from build123d import *

# Parameters (mm, degrees)
BOX063_W                   = 4
BOX063_H                   = 1.6
BOX063_DEPTH               = 0.6
CYLINDER043_R              = 1.5
CYLINDER043_DEPTH          = 0.6
CYLINDER042_R              = 2.2
CYLINDER042_DEPTH          = 0.6
BOX064_W                   = 3.6
BOX064_H                   = 0.8
BOX064_DEPTH               = 0.6
FUSION040_PLACEMENT_ANGLE  = 90
BOX061_W                   = 1.5
BOX061_H                   = 0.5
BOX061_DEPTH               = 3
BOX066_W                   = 1.5
BOX066_H                   = 0.5
BOX066_DEPTH               = 3
BOX060_W                   = 0.5
BOX060_H                   = 6
BOX060_DEPTH               = 1
BOX068_W                   = 52
BOX068_H                   = 6
BOX068_DEPTH               = 12
CYLINDER045_R              = 1.3
CYLINDER045_DEPTH          = 8
CYLINDER037_R              = 1.3
CYLINDER037_DEPTH          = 8
CYLINDER044_R              = 1.3
CYLINDER044_DEPTH          = 8
CYLINDER040_R              = 1.3
CYLINDER040_DEPTH          = 8
CYLINDER041_R              = 3
CYLINDER041_DEPTH          = 9.5
CYLINDER039_R              = 3
CYLINDER039_DEPTH          = 9.5
CYLINDER046_R              = 3
CYLINDER046_DEPTH          = 9.5
CYLINDER038_R              = 3
CYLINDER038_DEPTH          = 9.5
BOX069_W                   = 90
BOX069_H                   = 60
BOX069_DEPTH               = 1.6
BOX059_W                   = 1.5
BOX059_H                   = 5
BOX059_DEPTH               = 8.5
BOX070_W                   = 2
BOX070_H                   = 2
BOX070_DEPTH               = 2
BOX062_W                   = 2
BOX062_H                   = 2
BOX062_DEPTH               = 2
BOX065_W                   = 2
BOX065_H                   = 2
BOX065_DEPTH               = 2
BOX067_W                   = 2
BOX067_H                   = 2
BOX067_DEPTH               = 2
CHAMFER007_SIZE            = 0.6
CHAMFER007_PLACEMENT_ANGLE = 180


with BuildPart() as obj1:
    # Box063 → Box063 (new body)
    with BuildSketch(Plane(origin=(0, -0.8, 0), x_dir=(1, 0, 0), z_dir=(0, 0, 1))):
        with Locations((2, 0.8)):
            Rectangle(BOX063_W, BOX063_H)
    extrude(amount=BOX063_DEPTH)


with BuildPart() as zylinder042:
    # Cylinder043 → Cylinder043 (new body)
    with BuildSketch(Plane.XY):
        Circle(CYLINDER043_R)
    extrude(amount=CYLINDER043_DEPTH)


with BuildPart() as off:
    # Cylinder042 → Cylinder042 (new body)
    with BuildSketch(Plane.XY):
        Circle(CYLINDER042_R)
    extrude(amount=CYLINDER042_DEPTH)

    # Cut026: cut Zylinder042
    add(zylinder042.part, mode=Mode.SUBTRACT)

    # Cut023: cut obj1
    add(obj1.part, mode=Mode.SUBTRACT)


with BuildPart() as obj2:
    # Box064 → Box064 (new body)
    with BuildSketch(Plane(origin=(0, -0.4, 0), x_dir=(1, 0, 0), z_dir=(0, 0, 1))):
        with Locations((1.8, 0.4)):
            Rectangle(BOX064_W, BOX064_H)
    extrude(amount=BOX064_DEPTH)

    # Fusion040: union Off
    add(off.part)


with BuildPart() as obj2_1:
    # Fusion040 placement: moved
    add(obj2.part.moved(Location((-44.4, -1.5, 11))).rotate(Axis((-44.4, -1.5, 11), (0, -1, 0)), FUSION040_PLACEMENT_ANGLE))


with BuildPart() as obj3:
    # Box061 → Box061 (new body)
    with BuildSketch(Plane(origin=(-45, 1, 15), x_dir=(1, 0, 0), z_dir=(0, 0, 1))):
        with Locations((0.75, 0.25)):
            Rectangle(BOX061_W, BOX061_H)
    extrude(amount=BOX061_DEPTH)


with BuildPart() as obj4:
    # Box066 → Box066 (new body)
    with BuildSketch(Plane(origin=(-45, -4.5, 15), x_dir=(1, 0, 0), z_dir=(0, 0, 1))):
        with Locations((0.75, 0.25)):
            Rectangle(BOX066_W, BOX066_H)
    extrude(amount=BOX066_DEPTH)


with BuildPart() as obj5:
    # Box060 → Box060 (new body)
    with BuildSketch(Plane(origin=(-43.5, -4.5, 15), x_dir=(1, 0, 0), z_dir=(0, 0, 1))):
        with Locations((0.25, 3)):
            Rectangle(BOX060_W, BOX060_H)
    extrude(amount=BOX060_DEPTH)

    # Fusion038: union obj3, obj4
    add(obj3.part)
    add(obj4.part)


with BuildPart() as obj6:
    # Box068 → Box068 (new body)
    with BuildSketch(Plane(origin=(-36.38, 21.5, 6), x_dir=(1, 0, 0), z_dir=(0, 0, 1))):
        with Locations((26, 3)):
            Rectangle(BOX068_W, BOX068_H)
    extrude(amount=BOX068_DEPTH)


with BuildPart() as zylinder044:
    # Cylinder045 → Cylinder045 (new body)
    with BuildSketch(Plane(origin=(-39, 24.5, 0), x_dir=(1, 0, 0), z_dir=(0, 0, 1))):
        Circle(CYLINDER045_R)
    extrude(amount=CYLINDER045_DEPTH)


with BuildPart() as fusion064:
    # Cylinder037 → Cylinder037 (new body)
    with BuildSketch(Plane(origin=(-39, -24.5, 0), x_dir=(1, 0, 0), z_dir=(0, 0, 1))):
        Circle(CYLINDER037_R)
    extrude(amount=CYLINDER037_DEPTH)

    # Fusion064: union Zylinder044
    add(zylinder044.part)


with BuildPart() as fusion064_1:
    # Fusion064 placement: moved
    add(fusion064.part.moved(Location((58, 0, 0))))


with BuildPart() as zylinder043:
    # Cylinder044 → Cylinder044 (new body)
    with BuildSketch(Plane(origin=(-39, 24.5, 0), x_dir=(1, 0, 0), z_dir=(0, 0, 1))):
        Circle(CYLINDER044_R)
    extrude(amount=CYLINDER044_DEPTH)


with BuildPart() as obj7:
    # Cylinder040 → Cylinder040 (new body)
    with BuildSketch(Plane(origin=(-39, -24.5, 0), x_dir=(1, 0, 0), z_dir=(0, 0, 1))):
        Circle(CYLINDER040_R)
    extrude(amount=CYLINDER040_DEPTH)

    # Fusion070: union Zylinder043
    add(zylinder043.part)

    # Fusion069: union Fusion064
    add(fusion064_1.part)


with BuildPart() as obj7_1:
    # Fusion069 placement: moved
    add(obj7.part.moved(Location((0, 0, 5.6))))


with BuildPart() as zylinder040:
    # Cylinder041 → Cylinder041 (new body)
    with BuildSketch(Plane(origin=(-39, 24.5, 2), x_dir=(1, 0, 0), z_dir=(0, 0, 1))):
        Circle(CYLINDER041_R)
    extrude(amount=CYLINDER041_DEPTH)


with BuildPart() as fusion068:
    # Cylinder039 → Cylinder039 (new body)
    with BuildSketch(Plane(origin=(-39, -24.5, 2), x_dir=(1, 0, 0), z_dir=(0, 0, 1))):
        Circle(CYLINDER039_R)
    extrude(amount=CYLINDER039_DEPTH)

    # Fusion068: union Zylinder040
    add(zylinder040.part)


with BuildPart() as fusion068_1:
    # Fusion068 placement: moved
    add(fusion068.part.moved(Location((58, 0, 0))))


with BuildPart() as zylinder045:
    # Cylinder046 → Cylinder046 (new body)
    with BuildSketch(Plane(origin=(-39, 24.5, 2), x_dir=(1, 0, 0), z_dir=(0, 0, 1))):
        Circle(CYLINDER046_R)
    extrude(amount=CYLINDER046_DEPTH)


with BuildPart() as obj8:
    # Cylinder038 → Cylinder038 (new body)
    with BuildSketch(Plane(origin=(-39, -24.5, 2), x_dir=(1, 0, 0), z_dir=(0, 0, 1))):
        Circle(CYLINDER038_R)
    extrude(amount=CYLINDER038_DEPTH)

    # Fusion062: union Zylinder045
    add(zylinder045.part)

    # Fusion063: union Fusion068
    add(fusion068_1.part)


with BuildPart() as obj8_1:
    # Fusion063 placement: moved
    add(obj8.part.moved(Location((0, 0, 4.1))))

    # Cut022: cut obj7
    add(obj7_1.part, mode=Mode.SUBTRACT)


with BuildPart() as obj9:
    # Box069 → Box069 (new body)
    with BuildSketch(Plane(origin=(-45, -30, 15.5), x_dir=(1, 0, 0), z_dir=(0, 0, 1))):
        with Locations((45, 30)):
            Rectangle(BOX069_W, BOX069_H)
    extrude(amount=BOX069_DEPTH)

    # Fusion037: union obj8
    add(obj8_1.part)

    # Cut021: cut obj6
    add(obj6.part, mode=Mode.SUBTRACT)

    # Cut025: cut obj5
    add(obj5.part, mode=Mode.SUBTRACT)


with BuildPart() as deckel_mit_io_button:
    # Box059 → Box059 (new body)
    with BuildSketch(Plane(origin=(-45, -4, 7), x_dir=(1, 0, 0), z_dir=(0, 0, 1))):
        with Locations((0.75, 2.5)):
            Rectangle(BOX059_W, BOX059_H)
    extrude(amount=BOX059_DEPTH)

    # Fusion039: union obj9
    add(obj9.part)

    # Cut024: cut obj2
    add(obj2_1.part, mode=Mode.SUBTRACT)


with BuildPart() as obj10:
    # Box070 → Box070 (new body)
    with BuildSketch(Plane(origin=(41.3, -28.8, 14), x_dir=(1, 0, 0), z_dir=(0, 0, 1))):
        with Locations((1, 1)):
            Rectangle(BOX070_W, BOX070_H)
    extrude(amount=BOX070_DEPTH)


with BuildPart() as fusion066:
    # Box062 → Box062 (new body)
    with BuildSketch(Plane(origin=(41.3, 26.8, 14), x_dir=(1, 0, 0), z_dir=(0, 0, 1))):
        with Locations((1, 1)):
            Rectangle(BOX062_W, BOX062_H)
    extrude(amount=BOX062_DEPTH)

    # Fusion066: union obj10
    add(obj10.part)


with BuildPart() as fusion066_1:
    # Fusion066 placement: moved
    add(fusion066.part.moved(Location((-84.6, 0, 0))))


with BuildPart() as obj11:
    # Box065 → Box065 (new body)
    with BuildSketch(Plane(origin=(41.3, -28.8, 14), x_dir=(1, 0, 0), z_dir=(0, 0, 1))):
        with Locations((1, 1)):
            Rectangle(BOX065_W, BOX065_H)
    extrude(amount=BOX065_DEPTH)


with BuildPart() as obj12:
    # Box067 → Box067 (new body)
    with BuildSketch(Plane(origin=(41.3, 26.8, 14), x_dir=(1, 0, 0), z_dir=(0, 0, 1))):
        with Locations((1, 1)):
            Rectangle(BOX067_W, BOX067_H)
    extrude(amount=BOX067_DEPTH)

    # Fusion061: union obj11
    add(obj11.part)

    # Fusion065: union Fusion066
    add(fusion066_1.part)

    # Chamfer007
    chamfer007_edges = [obj12.edges().sort_by_distance(p)[0] for p in [
        (43.3, 27.8, 16),
        (42.3, 28.8, 16),
        (43.3, -27.8, 16),
        (42.3, -28.8, 16),
        (-43.3, 27.8, 16),
        (-42.3, 28.8, 16),
        (-43.3, -27.8, 16),
        (-42.3, -28.8, 16),
    ]]
    chamfer(chamfer007_edges, length=CHAMFER007_SIZE)


with BuildPart() as obj12_1:
    # Chamfer007 placement: moved
    add(obj12.part.moved(Location((0, 0, 29.5))).rotate(Axis((0, 0, 29.5), (1, 0, 0)), CHAMFER007_PLACEMENT_ANGLE))

    # Fusion067: union Deckel mit IO-Button
    add(deckel_mit_io_button.part)


with BuildPart() as obj12_2:
    # Fusion067 placement: moved
    add(obj12_1.part.moved(Location((0, 0, 14.75))))


solid = obj12_2.part
For this review, take the finished solid that the model builds, in its own axes (mm). A direction names the side the tool comes from. Round coordinates to 2 decimals unless told otherwise and drop trailing zeros. Write each loop counter-clockwise with the first axis right and the second up, starting at its lowest first coordinate (ties: lowest second). Pieces come first, ordered by that corner, then holes. Notation, with made-up numbers: (-31, -13) - (4, -13) arc R23 ccw to (4, 22) - close; hole circle Ø8 at (84.25, 70.25). An arc over 180 degrees is marked (long way). Write item = value, one per line. Start each with the question number.
1. Wall thickness on L1, parallel to X at y = -24.5, z = 26; L2, parallel to Y at x = 19, z = 25.5; L3, parallel to X at y = 24.5, z = 25.25: over which ranges is each line inside the solid? List them lowest first.
2. Consider section B-B on x = -39. State the section outline as (y, z) points, plus the area to 3 significant figures.
3. Draft analysis for pull direction Z (two halves, no side actions). For faces 5 (the face through (20, -26, 20.85)), 6 (the face through (-44.7, -1.41, 23.55)), 7 (the face through (-41.3, -28, 29)), state which applies: released by +Z, released by -Z, zero draft, split by the parting line, or undercut.
4. Consider section D-D on x = 36. State the section outline as (y, z) points, plus the area to 3 significant figures.
5. For pin 1 Ø0.6 at (x, z) = (42.5, 29.5) entering from -Y; pin 2 Ø1.1 at (x, y) = (42.5, 27.5) entering from -Z; pin 3 Ø1.5 at (y, z) = (-20, 23.5) entering from -X; pin 4 Ø2 at (x, y) = (19, 24.5) entering from -Z, all flat-tipped, find the tip position at first contact; note any pin that passes through.
6. For faces 1 (the face through (16, -24.4, 25.5)), 2 (the face through (-42, 26.8, 29)), 3 (the face through (-44.7, -1.45, 24.25)), 4 (the face through (41.3, -28, 29)), list the 3-axis set-ups (+Z, -Z, +X, -X, +Y, -Y) from which the entire face can be reached by the end or side of a thin tool; tool diameter is ignored.
7. Consider section C-C on y = -24.5. State the section outline as (x, z) points.
8. Consider section A-A on x = -21. State the section outline as (y, z) points.
Evaluation:
q1.L1 = -42 to -40.3, -37.7 to -36, 16 to 17.7, 20.3 to 22
q1.L2 = -27.5 to -25.8, -23.2 to -21.5, 21.5 to 23.2, 25.8 to 27.5
q1.L3 = -42 to -40.3, -37.7 to -36.38, 16 to 17.7, 20.3 to 22
q2.outline = (-30, 30.25) - (-27.5, 30.25) - (-27.5, 20.85) - (-25.8, 20.85) - (-25.8, 28.35) - (-23.2, 28.35) - (-23.2, 20.85) - (-21.5, 20.85) - (-21.5, 30.25) - (21.5, 30.25) - (21.5, 20.85) - (23.2, 20.85) - (23.2, 28.35) - (25.8, 28.35) - (25.8, 20.85) - (27.5, 20.85) - (27.5, 30.25) - (30, 30.25) - (30, 31.85) - (-30, 31.85) - close
q2.area = 170 mm2
q3.face_5 = released by -Z
q3.face_6 = undercut
q3.face_7 = zero draft
q4.outline = (-30, 30.25) - (30, 30.25) - (30, 31.85) - (-30, 31.85) - close
q4.area = 96.0 mm2
q5.pin_1 = -28.8
q5.pin_2 = 28.25
q5.pin_3 = through
q5.pin_4 = 28.35
q6.face_1 = -Z
q6.face_2 = -Z, -X
q6.face_3 = -X
q6.face_4 = -Z, +Y, -Y
q7.outline = (-45, 30.25) - (-42, 30.25) - (-42, 20.85) - (-40.3, 20.85) - (-40.3, 28.35) - (-37.7, 28.35) - (-37.7, 20.85) - (-36, 20.85) - (-36, 30.25) - (16, 30.25) - (16, 20.85) - (17.7, 20.85) - (17.7, 28.35) - (20.3, 28.35) - (20.3, 20.85) - (22, 20.85) - (22, 30.25) - (45, 30.25) - (45, 31.85) - (-45, 31.85) - close
q8.outline = (-30, 30.25) - (21.5, 30.25) - (21.5, 31.85) - (-30, 31.85) - close; (27.5, 30.25) - (30, 30.25) - (30, 31.85) - (27.5, 31.85) - close
